Work out the finished part from the listing and answer in its coordinate system (mm). A direction names the side the tool comes from. Round coordinates to 2 decimals unless told otherwise and drop trailing zeros. Write each loop counter-clockwise with the first axis right and the second up, starting at its lowest first coordinate (ties: lowest second). Pieces come first, ordered by that corner, then holes.
1. Find section A-A (y = 11). Write down the section's boundary in (x, z), and give its area (3 significant figures).
2. Find section D-D (x = 25). Write down the section's boundary in (y, z).
3. Straight lines are drawn through the part: probe 1 along X at (y, z) = (29.5, 11.5); probe 2 along Y at (x, z) = (23, 11); probe 3 along X at (y, z) = (11.5, 11.5). For each, find the intervals that lie inside material, in ascending order.
4. Flat-ended cylindrical pins translate along their axes: pin 1 Ø3 at (x, y) = (25.5, 19) entering from +Z; pin 2 Ø0.8 at (x, y) = (33, 56) entering from -Z; pin 3 Ø3 at (x, z) = (-2, 6.5) entering from +Y. Find the tip coordinate at first contact, or state that the pin passes through.
5. Find section B-B (x = 20). Write down the section's boundary in (y, z).
6. A tool of negligible diameter and unlimited length cuts with its end or side. For faces 1 (the face through (-2, 55, 12)), 2 (the face through (-2, 55, 2)), 3 (the face through (5, 64, 7)), 4 (the face through (16.22, 0.57, 0.6)), 5 (the face through (-2, 15.45, 7)), from which of +Z, -Z, +X, -X, +Y, -Y can it reach the whole face along a straight path? Write none if from no direction.
```python
from build123d import *

# Parameters (mm, degrees)
ESQUISSE1_W             = 34
ESQUISSE1_H             = 100.65
BOSS_EXTRU_1_DEPTH      = 12.5
ESQUISSE2_W             = 31
ESQUISSE2_H             = 97.65
ENL_V_MAT_EXTRU_1_DEPTH = 11
ESQUISSE5_R             = 2
BOSS_EXTRU_4_DEPTH      = 3
ESQUISSE6_R             = 1.3
BOSS_EXTRU_5_DEPTH      = 5.5
CONG_2_R                = 2
CONG_3_R                = 2
CONG_4_R                = 2
ESQUISSE7_W             = 7.5
ESQUISSE7_H             = 80
BOSS_EXTRU_6_DEPTH      = 1
ESQUISSE9_W             = 10
ESQUISSE9_H             = 80
BOSS_EXTRU_7_DEPTH      = 3
ESQUISSE10_W            = 4.6
ESQUISSE10_H            = 8.2
ESQUISSE10_W_2          = 4.5
ESQUISSE10_H_2          = 14
ENL_V_MAT_EXTRU_2_DEPTH = 3
ESQUISSE11_W            = 15.5
ESQUISSE11_H            = 4.6
ENL_V_MAT_EXTRU_3_DEPTH = 3


with BuildPart() as part:
    # Esquisse1 → Boss.-Extru.1 (new body)
    with BuildSketch(Plane.XY):
        with Locations((17, 50.325)):
            Rectangle(ESQUISSE1_W, ESQUISSE1_H)
    extrude(amount=BOSS_EXTRU_1_DEPTH)

    # Esquisse2 → Enlèv. mat.-Extru.1 (cut)
    with BuildSketch(Plane.XY.offset(12.5)):
        with Locations((17, 50.325)):
            Rectangle(ESQUISSE2_W, ESQUISSE2_H)
    extrude(amount=-ENL_V_MAT_EXTRU_1_DEPTH, mode=Mode.SUBTRACT)

    # Esquisse5 → Boss.-Extru.4 (add)
    with BuildSketch(Plane.XY.offset(1.5)):
        with Locations((5.5, 63.5)):
            Circle(ESQUISSE5_R)
        with Locations((28.5, 63.5)):
            Circle(ESQUISSE5_R)
        with Locations((5.5, 5.5)):
            Circle(ESQUISSE5_R)
        with Locations((28.5, 5.5)):
            Circle(ESQUISSE5_R)
    extrude(amount=BOSS_EXTRU_4_DEPTH)

    # Esquisse6 → Boss.-Extru.5 (add)
    with BuildSketch(Plane.XY.offset(1.5)):
        with Locations((5.5, 63.5)):
            Circle(ESQUISSE6_R)
        with Locations((28.5, 63.5)):
            Circle(ESQUISSE6_R)
        with Locations((5.5, 5.5)):
            Circle(ESQUISSE6_R)
        with Locations((28.5, 5.5)):
            Circle(ESQUISSE6_R)
    extrude(amount=BOSS_EXTRU_5_DEPTH)

    # Congé2
    cong_2_edges = [part.edges().sort_by_distance(p)[0] for p in [
        (34, 0, 6.25),
    ]]
    fillet(cong_2_edges, radius=CONG_2_R)

    # Congé3
    cong_3_edges = [part.edges().sort_by_distance(p)[0] for p in [
        (34, 100.65, 6.25),
    ]]
    fillet(cong_3_edges, radius=CONG_3_R)

    # Congé4
    cong_4_edges = [part.edges().sort_by_distance(p)[0] for p in [
        (16, 0, 0),
        (34, 50.325, 0),
        (33.414213562, 0.585786438, 0),
        (16, 100.65, 0),
        (33.414213562, 100.064213562, 0),
    ]]
    fillet(cong_4_edges, radius=CONG_4_R)

    # Esquisse7 → Boss.-Extru.6 (add)
    with BuildSketch(Plane.ZY):
        with Locations((7, 55.45)):
            Rectangle(ESQUISSE7_W, ESQUISSE7_H)
    extrude(amount=BOSS_EXTRU_6_DEPTH)

    # Esquisse9 → Boss.-Extru.7 (add)
    with BuildSketch(Plane.ZY.offset(1)):
        with Locations((7, 55.45)):
            Rectangle(ESQUISSE9_W, ESQUISSE9_H)
    extrude(amount=BOSS_EXTRU_7_DEPTH)

    # Esquisse10 → Enlèv. mat.-Extru.2 (cut)
    with BuildSketch(Plane.ZY.offset(-32.5)):
        with Locations((7.8, 56)):
            Rectangle(ESQUISSE10_W, ESQUISSE10_H)
        with Locations((7.8, 43.4)):
            Rectangle(ESQUISSE10_W, ESQUISSE10_H)
        with Locations((7.75, 14.4)):
            Rectangle(ESQUISSE10_W_2, ESQUISSE10_H_2)
    extrude(amount=-ENL_V_MAT_EXTRU_2_DEPTH, mode=Mode.SUBTRACT)

    # Esquisse11 → Enlèv. mat.-Extru.3 (cut)
    with BuildSketch(Plane(origin=(0, 1.5, 0), x_dir=(1, 0, 0), z_dir=(0, 1, 0))):
        with Locations((14.724178104, -7.8)):
            Rectangle(ESQUISSE11_W, ESQUISSE11_H)
    extrude(amount=-ENL_V_MAT_EXTRU_3_DEPTH, mode=Mode.SUBTRACT)


solid = part.part
```
Worked answers:
1. outline: (0, 0) - (32, 0) arc R2 ccw to (34, 2) - (34, 5.5) - (32.5, 5.5) - (32.5, 1.5) - (1.5, 1.5) - (1.5, 12.5) - (0, 12.5) - close; (32.5, 10) - (34, 10) - (34, 12.5) - (32.5, 12.5) - close
1. area: 76.4 mm2
2. outline: (0, 2) arc R2 ccw to (2, 0) - (98.65, 0) arc R2 ccw to (100.65, 2) - (100.65, 12.5) - (99.15, 12.5) - (99.15, 1.5) - (1.5, 1.5) - (1.5, 12.5) - (0, 12.5) - close
3. probe 1: x = -4 to -1, 0 to 1.5, 32.5 to 34
3. probe 2: y = 0 to 1.5, 99.15 to 100.65
3. probe 3: x = 0 to 1.5, 32.5 to 34
4. pin 1: stops at z = 1.5
4. pin 2: stops at z = 0.09
4. pin 3: stops at y = 95.45
5. outline: (0, 2) arc R2 ccw to (2, 0) - (98.65, 0) arc R2 ccw to (100.65, 2) - (100.65, 12.5) - (99.15, 12.5) - (99.15, 1.5) - (1.5, 1.5) - (1.5, 5.5) - (0, 5.5) - close; (0, 10.1) - (1.5, 10.1) - (1.5, 12.5) - (0, 12.5) - close
6. face 1: +Z, -X, +Y, -Y
6. face 2: -Z, -X, +Y, -Y
6. face 3: +Z
6. face 4: -Z, +X, -X, -Y
6. face 5: +Z, -Z, -X, -Y
